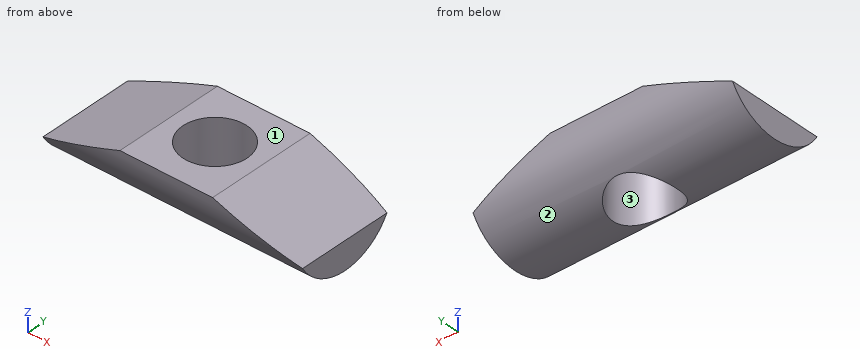
from build123d import *

# Parameters (mm, degrees)
EXTRUDE1_START           = -14
SKETCH1_R                = 6
EXTRUDE1_DEPTH           = 28
EXTRUDE2_DEPTH           = 20
EXTRUDE2_DEPTH_BACK      = 20
F_5_16_24_TAPPED_HOLE1_D = 6.9088


with BuildPart() as part:
    # Sketch1 → Extrude1 (new body)
    with BuildSketch(Plane(origin=(0, 0, 0), x_dir=(0, 0, -1), z_dir=(1, 0, 0)).offset(EXTRUDE1_START)):
        Circle(SKETCH1_R)
    extrude(amount=EXTRUDE1_DEPTH)

    # Sketch2 → Extrude2 (cut, two sides)
    with BuildSketch(Plane(origin=(0, 0, 0), x_dir=(1, 0, 0), z_dir=(0, 1, 0))) as extrude2_sk:
        Polygon((-5, -0.275732108), (5, -0.275732108), (14, 3), (25.458166387, 3), (25.458166387, -16.52435343), (-25.590688577, -16.52435343), (-25.590688577, 3), (-14, 3), align=None)
    extrude(amount=EXTRUDE2_DEPTH, mode=Mode.SUBTRACT)
    extrude(extrude2_sk.sketch, amount=-EXTRUDE2_DEPTH_BACK, mode=Mode.SUBTRACT)

    # 5_16-24 Tapped Hole1 (through all)
    with Locations(Plane.XY.offset(0.275732108)):
        with Locations((0, 0)):
            Hole(F_5_16_24_TAPPED_HOLE1_D / 2)


solid = part.part
Work out the finished part from the listing and answer in its coordinate system (mm). Face numbers are marked on the shaded views. Coordinates: 2 decimals unless noted, no trailing zeros. Write each loop counter-clockwise with the first axis right and the second up, starting at its lowest first coordinate (ties: lowest second). Pieces come first, ordered by that corner, then holes. Notation, with made-up numbers: (71.25, 23.5) - (128.25, 23.5) arc R23 ccw to (128.25, 33.5) - close; hole circle Ø11 at (-31.75, 88.25). An arc over 180 degrees is marked (long way). One line per question, with ' | ' between items.
1) Find section D-D, the plane y = 2.5. Determine the outline of the cut face in (x, z).
Checks:
outline: (-14, -5.45) - (-2.38, -5.45) - (-2.38, 0.28) - (-5, 0.28) - (-14, -3) - close; (2.38, -5.45) - (14, -5.45) - (14, -3) - (5, 0.28) - (2.38, 0.28) - close
2) Consider probe 1 along X at (y, z) = (0, -3.5); probe 2 along X at (y, z) = (2, -4.5); probe 3 along Y at (x, z) = (-2.25, -0.25). Determine where each line is inside the solid, lowest interval first. Write a range as [from, to].
Checks:
probe 1: [-14, -3.45], [3.45, 14] | probe 2: [-14, -2.82], [2.82, 14] | probe 3: [-5.99, -2.62], [2.62, 5.99]
3) Find section C-C, the plane x = 0. Determine the outline of the cut face in (y, z), and give its area (3 significant figures).
Checks:
outline: (-5.99, 0.28) arc R6 ccw to (-3.45, -4.91) - (-3.45, 0.28) - close; (3.45, -4.91) arc R6 ccw to (5.99, 0.28) - (3.45, 0.28) - close | area: 18.9 mm2
4) Find section A-A, the plane y = 0. Determine the outline of the cut face in (x, z).
Checks:
outline: (-14, -6) - (-3.45, -6) - (-3.45, 0.28) - (-5, 0.28) - (-14, -3) - close; (3.45, -6) - (14, -6) - (14, -3) - (5, 0.28) - (3.45, 0.28) - close
5) Find section B-B, the plane z = -1.75. Determine the outline of the cut face in (x, y).
Checks:
outline: (-10.57, -5.74) - (10.57, -5.74) - (10.57, 5.74) - (-10.57, 5.74) - close; hole circle Ø6.91 at (0, 0)
6) The mould has two halves that part along Y. Classify the marked faces 1, 2 and 3: +Y half, -Y half, draft (parallel to the pull), parting line (faces both ways), or undercut.
Checks:
face 1: draft | face 2: parting line | face 3: undercut
7) Flat-ended cylindrical pins translate along their axes: P1, Ø1.5, axis at x = 1.5, z = -3, coming from the -Y side; P2, Ø2, axis at x = -6.5, y = -2, coming from the +Z side. Find the tip coordinate at first contact, or state that the pin passes through.
Checks:
P1: y = -5.56 | P2: z = 0.09
